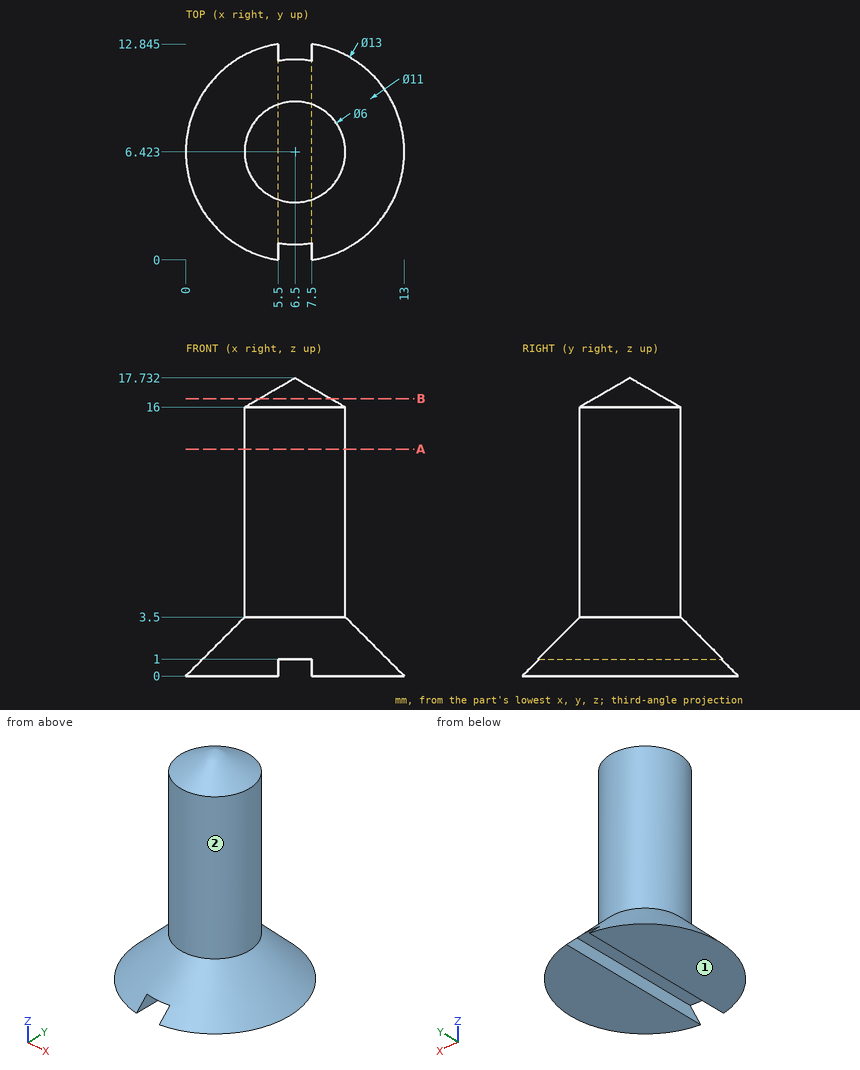
Drawing for the job (mm, zero at the part's lowest x, y, z). A direction names the side the tool comes from. Round coordinates to 2 decimals unless told otherwise and drop trailing zeros. Loops run counter-clockwise (first coordinate to the right, second up) from the corner with the lowest first, then second, coordinate; pieces in that order, holes last. Notation, with made-up numbers: (15.5, -34) - (26.5, -34) arc R16 cw to (26.5, -29) - close; hole circle Ø11 at (48.25, 9.25). An arc over 180 degrees is marked (long way). Write each question's results on one line, items separated by ' | '.
(1) Wall check: L1, parallel to X at y = 6.25, z = 13 (1 decimal); L2, parallel to X at y = 7.5, z = 5; L3, parallel to Z at x = 5.25, y = 5.5 (1 decimal). Give the ranges that are in metal, low to high.
Answer below:
L1: x = 3.5 to 9.5 | L2: x = 3.7 to 9.3 | L3: z = 0 to 16.8
(2) Saw through at A-A, the plane z = 13.5. List the corners of the cut face in (x, y), then the cut area to 3 significant figures.
Answer below:
outline: circle Ø6 at (6.5, 6.42) | area: 28.3 mm^2
(3) Pin check, flat tips, straight feed: pin 1 (3 mm diameter, centred on x = 5, z = 9.5, fed in from -Y); pin 2 (5 mm diameter, centred on y = 5.5, z = 2, fed in from -X); pin 3 (1 mm diameter, centred on x = 6, y = 9.5, fed in from +Z); pin 4 (2 mm diameter, centred on y = 1.5, z = 14, fed in from -X). Stop position of each tip, or through.
Answer below:
pin 1: stops at y = 3.42 | pin 2: stops at x = 0 | pin 3: stops at z = 16.22 | pin 4: passes through
(4) Saw through at B-B, the plane z = 16.5. List the corners of the cut face in (x, y).
Answer below:
outline: circle Ø4.27 at (6.5, 6.42)
(5) 3-axis set-ups, long thin cutter, end or side, ignore diameter. For the marked faces 1 and 2: which of +Z, -Z, +X, -X, +Y, -Y reach the whole face in a straight line?
Answer below:
face 1: -Z, +X, -X, +Y, -Y | face 2: +Z
